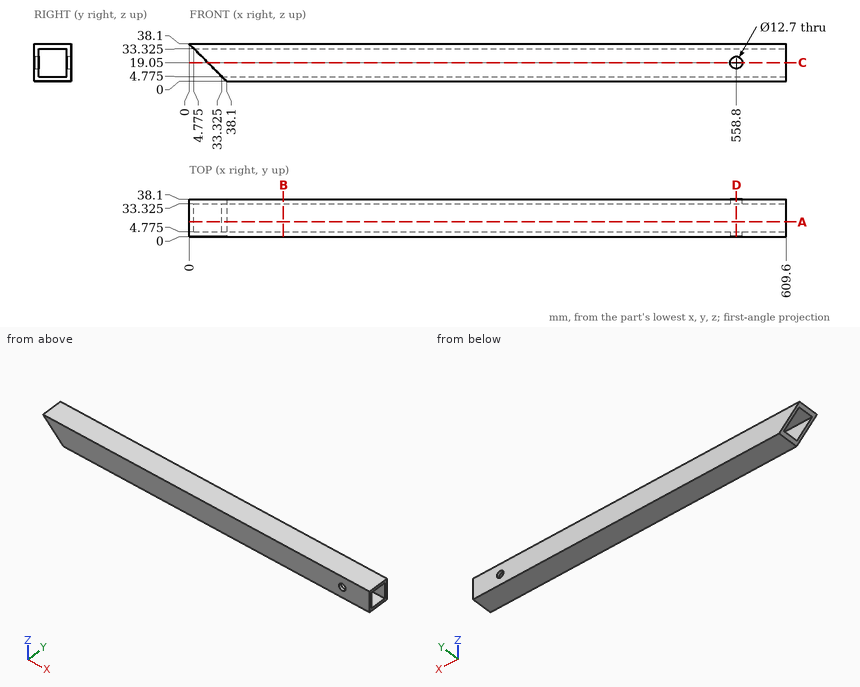
Could you check a few things on this drawing? It's one solid part, dimensions in mm from its lowest x, y, z. Give positions to 0.01 mm unless a question says otherwise; leave off trailing zeros. Write each loop counter-clockwise with the first axis right and the second up, starting at its lowest first coordinate (ties: lowest second). Pieces come first, ordered by that corner, then holes. Notation, with made-up numbers: (46.25, -0.75) - (63.25, -0.75) arc R33 ccw to (63.25, 36.25) - close; hole circle Ø5 at (2.5, 48). An arc over 180 degrees is marked (long way). Use CSV: the item, a comma, the result in double quotes. Start each with the question number.
Item 1: I want a section at B-B, the plane x = 96. Please give me the cut outline in (y, z) (1 decimal).
Item 2: I want a section at D-D, the plane x = 558.8. Please give me the cut outline in (y, z) (1 decimal).
Item 3: I want a section at A-A, the plane y = 15. Please give me the cut outline in (x, z) (1 decimal), then the cut area to 3 significant figures.
Item 4: If I drill on line 1 along Y through (x, z) = (435, 26.5) (1 decimal); line 2 along Z through (x, y) = (558.8, 36.15), over which ranges is the centre line in solid material (lowest first)?
Item 5: I want a section at C-C, the plane z = 19.05. Give the number of separate pieces and of enclosed holes in the cut face, then the cut area to 3 significant figures.
Findings:
1,outline,"(0, 0) - (38.1, 0) - (38.1, 38.1) - (0, 38.1) - close; hole (4.8, 4.8) - (33.3, 4.8) - (33.3, 33.3) - (4.8, 33.3) - close"
2,outline,"(0, 0) - (38.1, 0) - (38.1, 12.7) - (33.3, 12.7) - (33.3, 4.8) - (4.8, 4.8) - (4.8, 12.7) - (0, 12.7) - close; (0, 25.4) - (4.8, 25.4) - (4.8, 33.3) - (33.3, 33.3) - (33.3, 25.4) - (38.1, 25.4) - (38.1, 38.1) - (0, 38.1) - close"
3,outline,"(0, 38.1) - (4.8, 33.3) - (609.6, 33.3) - (609.6, 38.1) - close; (33.3, 4.8) - (38.1, 0) - (609.6, 0) - (609.6, 4.8) - close"
3,area,"5,640 mm2"
4,line 1,"y = 0 to 4.8, 33.3 to 38.1"
4,line 2,"z = 0 to 12.7, 25.4 to 38.1"
5,separate pieces,"4"
5,enclosed holes,"0"
5,area,"5,520 mm2"
